```python
from build123d import *

# Parameters (mm, degrees)
IZIM1_R                     = 7.5
Y_KSEKLIK_EKSTR_ZYON1_DEPTH = 15
IZIM2_R                     = 7.5
IZIM2_R_2                   = 4.2
Y_KSEKLIK_EKSTR_ZYON2_DEPTH = 30
IZIM3_R                     = 1.5
KES_EKSTR_ZYON1_DEPTH       = 10


with BuildPart() as part:
    # Çizim1 → Yükseklik-Ekstrüzyon1 (new body)
    with BuildSketch(Plane(origin=(0, 0, 0), x_dir=(1, 0, 0), z_dir=(0, 1, 0))):
        with Locations(Location((0, 0, 0), (0, 0, 270))):
            Circle(IZIM1_R)
        with BuildLine():
            Line((-1.65, 2.2), (1.65, 2.2))
            ThreePointArc((1.65, 2.2), (0, -2.75), (-1.65, 2.2))
        make_face(mode=Mode.SUBTRACT)
    extrude(amount=Y_KSEKLIK_EKSTR_ZYON1_DEPTH)

    # Çizim2 → Yükseklik-Ekstrüzyon2 (add)
    with BuildSketch(Plane(origin=(0, 15, 0), x_dir=(1, 0, 0), z_dir=(0, 1, 0))):
        with Locations(Location((0, 0, 0), (0, 0, 270))):
            Circle(IZIM2_R)
        with Locations(Location((0, 0, 0), (0, 0, 270))):
            Circle(IZIM2_R_2, mode=Mode.SUBTRACT)
    extrude(amount=Y_KSEKLIK_EKSTR_ZYON2_DEPTH)

    # Çizim3 → Kes-Ekstrüzyon1 (cut)
    with BuildSketch(Plane.XY):
        with Locations(Location((0, 40, 0), (0, 0, 90))):
            Circle(IZIM3_R)
        with Locations(Location((0, 35, 0), (0, 0, 90))):
            Circle(IZIM3_R)
        with Locations(Location((0, 30, 0), (0, 0, 90))):
            Circle(IZIM3_R)
        with Locations((0, 10)):
            Circle(IZIM3_R)
        with Locations((0, 5)):
            Circle(IZIM3_R)
    extrude(amount=-KES_EKSTR_ZYON1_DEPTH, mode=Mode.SUBTRACT)


solid = part.part
```
Source: CAD feature listing. Evaluate the final solid. Frame: model axes, mm. A direction names the side the tool comes from. Coordinates: 2 decimals unless noted, no trailing zeros. Order: outer loops, then holes, each group sorted by start corner. A loop starts at its lowest first (then second) coordinate and runs counter-clockwise, first axis right, second up. Notation, with made-up numbers: (-3.5, 57) - (50.5, 57) arc R20 cw to (50.5, 68) - close; hole circle Ø10 at (8.25, 21.25). An arc over 180 degrees is marked (long way). One line per item, written item: value.
1) Mould query, pull axis Z, two halves, no side actions, for faces 1 (the face through (1.262, 29.79, 4.006)), 2 (the face through (0.1, 7.4, 2.75)), 3 (the face through (0.33, 22.185, -7.493)), 4 (the face through (-1.487, 39.805, -5.686)). Classes: released by +Z, released by -Z, zero draft, split by the parting line, or undercut.
Computed values:
face 1: undercut
face 2: undercut
face 3: split by the parting line
face 4: zero draft
2) Reachability of faces 5 (the face through (-1.487, 34.805, -5.686)), 6 (the face through (0, 0, 3)), 7 (the face through (-3.2, 45, 3.2)), 8 (the face through (0, 7, -2.2)), 9 (the face through (-3, 15, 1)) from +Z, -Z, +X, -X, +Y, -Y: full face, straight path, thin tool, end or side. Return the list, or none.
Computed values:
face 5: -Z
face 6: +Z, -Z, +X, -X, -Y
face 7: +Z, -Z, +X, -X, +Y
face 8: +Y, -Y
face 9: +Y
3) Cut plane A-A on z = 0. Output: boundary loops of the cut face in (x, y).
Computed values:
outline: (-7.5, 0) - (-2.75, 0) - (-2.75, 15) - (-4.2, 15) - (-4.2, 45) - (-7.5, 45) - close; (2.75, 0) - (7.5, 0) - (7.5, 45) - (4.2, 45) - (4.2, 15) - (2.75, 15) - close
4) Contact query for flat-ended pins moving along their axis: pin 1 (1.8 mm diameter, centred on x = 0, y = 40, fed in from -Z); pin 2 (8 mm diameter, centred on y = 32, z = -5.5, fed in from -X); pin 3 (5 mm diameter, centred on x = 0, z = 0, fed in from +Y). Output: stop coordinate, or through.
Computed values:
pin 1: stops at z = 4.1
pin 2: stops at x = -7.35
pin 3: stops at y = 15
5) Ray query, line 1 (Y direction, x = 0.75, z = -5); line 2 (X direction, y = 8.5, z = 0); line 3 (Z direction, x = 0, y = 29). Return the intervals inside material, ascending. Write a range as [from, to].
Computed values:
line 1: y = [0, 3.7], [6.3, 8.7], [11.3, 28.7], [31.3, 33.7], [36.3, 38.7], [41.3, 45]
line 2: x = [-7.5, -2.75], [2.75, 7.5]
line 3: z = [4.2, 7.5]
6) Cut plane B-B on x = 0. State how many separate pieces and enclosed holes the cut face has, plus the area to 3 significant figures.
Computed values:
separate pieces: 7
enclosed holes: 0
area: 287 mm^2
7) Cut plane C-C on z = -6.25. Output: boundary loops of the cut face in (x, y), plus the area to 3 significant figures.
Computed values:
outline: (-4.15, 0) - (4.15, 0) - (4.15, 45) - (-4.15, 45) - close; hole circle Ø3 at (0, 5); hole circle Ø3 at (0, 10); hole circle Ø3 at (0, 30); hole circle Ø3 at (0, 35); hole circle Ø3 at (0, 40)
area: 338 mm^2
8) Cut plane D-D on y = 7. Output: boundary loops of the cut face in (x, z).
Computed values:
outline: circle Ø15 at (0, 0); hole (-1.65, -2.2) - (1.65, -2.2) arc R2.75 ccw (long way) to start
